```python
from build123d import *

# Parameters (mm, degrees)
F0_R     = 2.921
F1_DEPTH = 19.05
F2_R     = 7.14375
F2_R_2   = 2.921
F3_DEPTH = 3.175
F4_R     = 0.79375
F5_DEPTH = 19.051
F8_R     = 0.508


# Not quite as in the source:
# - a feature names something its author has since deleted; it is built from what else it names


with BuildPart() as f1:
    # F0 (on Front) → F1 (new body)
    with BuildSketch(Plane.XZ):
        Circle(F0_R)
    extrude(amount=-F1_DEPTH)

    # F2 (on face) → F3 (join)
    with BuildSketch(Plane(origin=(0, 19.05, 0), x_dir=(-1, 0, 0), z_dir=(0, 1, 0))):
        Circle(F2_R)
        Circle(F2_R_2, mode=Mode.SUBTRACT)
    extrude(amount=-F3_DEPTH)

    # F4 (on face) → F5 (cut, through all)
    with BuildSketch(Plane.XZ):
        Circle(F4_R)
    extrude(amount=-F5_DEPTH, mode=Mode.SUBTRACT)

    # F6 (on Right) → F7 (revolve, cut)
    with BuildSketch(Plane.YZ):
        with BuildLine():
            ThreePointArc((19.0884582698, 0), (18.6124325104, -3.7323455074), (17.335280776, -7.2715384886))
            Line((17.335280776, -7.2715384886), (21.6284582698, -7.2715384886))
            Line((21.6284582698, -7.2715384886), (21.6284582698, 0))
            Line((21.6284582698, 0), (19.0884582698, 0))
        make_face()
    revolve(axis=Axis((0, 12.9899214953, 0), (0, 1, 0)), mode=Mode.SUBTRACT)

    # F8
    f8_edges = [f1.edges().sort_by_distance(p)[0] for p in [
        (5.051394, 17.397311, 5.051394),
        (-5.051394, 17.397311, -5.051394),
    ]]
    fillet(f8_edges, radius=F8_R)


solid = f1.part
```
Could you check a few things on this model? Use its own coordinates, in mm. Give positions to 0.01 mm unless a question says otherwise; leave off trailing zeros. Order: outer loops, then holes, each group sorted by start corner. A loop starts at its lowest first (then second) coordinate and runs counter-clockwise, first axis right, second up.
Q1. If I drill on line 1 along Z through (x, y) = (0, 6.75); line 2 along Z through (x, y) = (-0.5, 13.75); line 3 along Y through (x, z) = (1.5, -3.75) (3 decimals), over which ranges is the centre line in solid material (lowest first)?
Q2. We'd pull the mould along X, two halves only. Please class faces 1 (the cylindrical face through (-0.172, 9.392, -0.775)), 2 (the cylindrical face through (-0.633, 7.826, -2.852)), 3 (the flat face through (0.1, 15.875, -3.1)): +X half, -X half, draft (parallel to the pull), parting line (faces both ways), or undercut.
Q3. Suppose I cut it at A-A, the plane y = 5. Write out the boundary of the cut face in (x, z), and give its area (3 significant figures).
Q4. I'm going to push flat-ended pins straight in: P1, Ø1, axis at x = 4, y = 10.5, coming from the +Z side; P2, Ø6, axis at y = 5, z = 1, coming from the +X side; P3, Ø1.5, axis at x = 2, y = 10, coming from the +Z side; P4, Ø3, axis at x = -1.5, y = 11, coming from the -Z side. Where does each tip first touch, or does it pass through?
Solution:
1. line 1: z = -2.92 to -0.79, 0.79 to 2.92
1. line 2: z = -2.88 to -0.62, 0.62 to 2.88
1. line 3: y = 15.875 to 18.536
2. face 1: undercut
2. face 2: parting line
2. face 3: draft
3. outline: circle Ø5.84 at (0, 0); hole circle Ø1.59 at (0, 0)
3. area: 24.8 mm2
4. P1: passes through
4. P2: stops at x = 2.92
4. P3: stops at z = 2.64
4. P4: stops at z = -2.92
